Here's how the part is built. I have some questions about the finished solid (model axes, mm). A direction names the side the tool comes from. Give positions to 0.01 mm unless a question says otherwise; leave off trailing zeros. Write each loop counter-clockwise with the first axis right and the second up, starting at its lowest first coordinate (ties: lowest second). Pieces come first, ordered by that corner, then holes. Notation, with made-up numbers: (-25, 72) -> (25, 72) arc R17 cw to (25, 94) -> close; hole circle Ø4 at (6, 42). An arc over 180 degrees is marked (long way). Return JSON: item names as keys, results as strings.
from build123d import *

# Parameters (mm, degrees)
F0_R     = 6
F1_DEPTH = 60
F2_R     = 4.05
F3_DEPTH = 16.002
F4_R     = 0.889
F5_DEPTH = 120.001
F6_W     = 1.651
F6_H     = 1.27


with BuildPart() as f1:
    # F0 (on Front) → F1 (new body, symmetric)
    with BuildSketch(Plane.XZ):
        Circle(F0_R)
    extrude(amount=F1_DEPTH, both=True)

    # F2 (on face) → F3 (cut)
    with BuildSketch(Plane.XZ.offset(60)):
        Circle(F2_R)
    extrude(amount=-F3_DEPTH, mode=Mode.SUBTRACT)

    # F4 (on face) → F5 (cut, through all)
    with BuildSketch(Plane(origin=(0, 60, 0), x_dir=(-1, 0, 0), z_dir=(0, 1, 0))):
        Circle(F4_R)
    extrude(amount=-F5_DEPTH, mode=Mode.SUBTRACT)

    # F6 (on Top) → F7 (revolve, cut)
    with BuildSketch(Plane.XY):
        with Locations((-4.6665, -59.365)):
            Rectangle(F6_W, F6_H)
    revolve(axis=Axis((0, -59.477242, 0), (0, 1, 0)), mode=Mode.SUBTRACT)


solid = f1.part
1. For pin 1 Ø1.4 at (x, z) = (0, 0) entering from +Y; pin 2 Ø1.5 at (y, z) = (10, -2) entering from -X; pin 3 Ø6.5 at (x, z) = (0, 0) entering from -Y; pin 4 Ø1.5 at (x, y) = (-4.5, 3.5) entering from -Z, each with a flat end and sliding along its axis, tell me the tip position at first contact or that it passes through.
Taken from the geometry:
{"pin 1": "passes through", "pin 2": "stops at x = -5.87", "pin 3": "stops at y = -44", "pin 4": "stops at z = -4.68"}
2. Which directions (+Z, -Z, +X, -X, +Y, -Y) give clear straight access to the entire face, cutting with the end or side of a thin tool? Please do faces 5 (the face through (2, -58.73, -4)), 6 (the face through (3, -60, -5)).
Taken from the geometry:
{"face 5": "-Y", "face 6": "+Z, -Z, +X, -X, -Y"}
3. Suppose I cut it at A-A, the plane y = 47.5. List the corners of the cut face in (x, z) for me, and give its area (3 significant figures).
Taken from the geometry:
{"outline": "circle Ø12 at (0, 0); hole circle Ø1.78 at (0, 0)", "area": "111 mm²"}
4. If I drill on line 1 (Z direction, x = 0, y = 33.5); line 2 (Z direction, x = 0, y = -58.95); line 3 (Y direction, x = 2.75, z = -2), over which ranges is the centre line in solid material (lowest first)? Write a range as [from, to].
Taken from the geometry:
{"line 1": "z = [-6, -0.89], [0.89, 6]", "line 2": "z = [-6, -5.49], [5.49, 6]", "line 3": "y = [-44, 60]"}
5. Suppose I cut it at B-B, the plane x = -2.75. List the corners of the cut face in (y, z) for me, and give its area (3 significant figures).
Taken from the geometry:
{"outline": "(-60, -5.33) -> (60, -5.33) -> (60, 5.33) -> (-60, 5.33) -> (-60, 4.75) -> (-58.73, 4.75) -> (-58.73, 2.97) -> (-44, 2.97) -> (-44, -2.97) -> (-58.73, -2.97) -> (-58.73, -4.75) -> (-60, -4.75) -> close", "area": "1,180 mm²"}
6. If we mould it in two halves opening along X, with no side actions, what happens to faces 1 (the face through (1.2, 60, 0.1)), 2 (the face through (-6, -1, 0)), 3 (the face through (1, -43.998, -1)), 4 (the face through (-0.878, -51.467, -3.954))? For each: released by +X, released by -X, zero draft, split by the parting line, or undercut.
Taken from the geometry:
{"face 1": "zero draft", "face 2": "split by the parting line", "face 3": "undercut", "face 4": "undercut"}
